Part model, mm, in its own coordinate system. A direction names the side the tool comes from. Coordinates: 2 decimals unless noted, no trailing zeros. Order: outer loops, then holes, each group sorted by start corner. A loop starts at its lowest first (then second) coordinate and runs counter-clockwise, first axis right, second up.
from build123d import *

# Parameters (mm, degrees)
F0_W     = 100.1865565777
F0_H     = 92.3875570297
F1_DEPTH = 311.15
F2_R     = 31.3492715111
F3_DEPTH = 339.6968106
F3_TAPER = -23


# Not quite as in the source:
# - an extrude ends at something that could not be found from the text; its depth is read off the source's solid


with BuildPart() as f1:
    # F0 (on Top) → F1 (new body)
    with BuildSketch(Plane.XY):
        Rectangle(F0_W, F0_H)
    extrude(amount=F1_DEPTH)

    # F2 (on face) → F3 (join, through all)
    with BuildSketch(Plane.XY.offset(311.15)):
        Circle(F2_R)
    extrude(amount=F3_DEPTH, taper=F3_TAPER)


solid = f1.part
Q1. Wall check: line 1 along X through (y, z) = (5, 235.5); line 2 along Y through (x, z) = (17, 108); line 3 along Z through (x, y) = (-13.5, -42.5). Give the ranges that are in metal, low to high.
Results list:
line 1: x = -50.09 to 50.09
line 2: y = -46.19 to 46.19
line 3: z = 0 to 311.15, 342.35 to 650.85
Q2. Which spindle directions (+Z, -Z, +X, -X, +Y, -Y) get a long thin tool onto all of the face, cutting with end or side? Do faces 4 (the face through (-50.093, -1, 153)), 5 (the face through (-19.17, -86.33, 445.63)), 6 (the face through (-1, 1, 0)), 7 (the face through (50.093, -1, 153)), 8 (the face through (-1, 46.194, 153)). Say none if no direction does.
Results list:
face 4: -Z, -X, +Y, -Y
face 5: none
face 6: -Z, +X, -X, +Y, -Y
face 7: -Z, +X, +Y, -Y
face 8: -Z, +X, -X, +Y
Q3. Pin check, flat tips, straight feed: pin 1 Ø10 at (x, z) = (129, 582.5) entering from -Y; pin 2 Ø1 at (x, y) = (111.5, -31.5) entering from -Z; pin 3 Ø1 at (x, z) = (-79.5, 467.5) entering from -Y. Stop position of each tip, or through.
Results list:
pin 1: stops at y = -79.01
pin 2: stops at z = 509.08
pin 3: stops at y = -57.6
Q4. Cut at B-B on z = 193.5. Write the cut outline in (x, y).
Results list:
outline: (-50.09, -46.19) - (50.09, -46.19) - (50.09, 46.19) - (-50.09, 46.19) - close
Q5. Cut at C-C on z = 446. Write the cut outline in (x, y), and give its area (3 significant figures).
Results list:
outline: circle Ø177.18 at (0, 0)
area: 24,700 mm2
Q6. Mould opens along Z. For faces 1 (the face through (-1, -46.194, 153)), 2 (the face through (-2, 2, 650.847)), 3 (the face through (-12, 31, 311.15)) say: pulls with the +Z half, pulls with the -Z half, needs draft (parallel to the pull), parting line crosses it, or undercut.
Results list:
face 1: needs draft
face 2: pulls with the +Z half
face 3: undercut
Q7. Cut at A-A on x = 0. Write the cut outline in (y, z), and give its area (3 significant figures).
Results list:
outline: (-175.54, 650.85) - (-31.35, 311.15) - (-46.19, 311.15) - (-46.19, 0) - (46.19, 0) - (46.19, 311.15) - (31.35, 311.15) - (175.54, 650.85) - close
area: 99,000 mm2
